```python
from build123d import *

# Parameters (mm, degrees)
ESQUISSE1_W                                  = 250
ESQUISSE1_H                                  = 400
BOSS_EXTRU_1_DEPTH                           = 10
ESQUISSE2_R                                  = 13.5
ENL_V_MAT_EXTRU_1_DEPTH                      = 237.061432682
CHANFREIN1_SIZE                              = 3
TROU_TARAUD_M51_D                            = 4.2
TROUS_DE_CENTRAGE_4_0MM2_D                   = 4
TROUS_DE_CENTRAGE_6_0MM2_D                   = 6
D_GAGEMENT_M41_D                             = 4.5
R_P_TITION_LIN_AIRE1_COUNT                   = 2
R_P_TITION_LIN_AIRE1_PITCH                   = 120
R_P_TITION_LIN_AIRE1_COUNT_DIR2              = 2
R_P_TITION_LIN_AIRE1_PITCH_DIR2              = 340
R_P_TITION_LIN_AIRE2_COUNT                   = 2
R_P_TITION_LIN_AIRE2_PITCH                   = 30
R_P_TITION_LIN_AIRE2_COUNT_DIR2              = 2
R_P_TITION_LIN_AIRE2_PITCH_DIR2              = 25
R_P_TITION_LIN_AIRE3_COUNT                   = 2
R_P_TITION_LIN_AIRE3_PITCH                   = 120
R_P_TITION_LIN_AIRE3_COUNT_DIR2              = 2
R_P_TITION_LIN_AIRE3_PITCH_DIR2              = 340
D_GAGEMENT_M42_D                             = 4.5
CHAMBRAGE_POUR_VIS_T_TE_RONDE_BOMB_2_A_COUNT = 2
CHAMBRAGE_POUR_VIS_T_TE_RONDE_BOMB_2_A_PITCH = 180
CHAMBRAGE_POUR_VIS_T_TE_RONDE_BOMB_3_COUNT   = 2
CHAMBRAGE_POUR_VIS_T_TE_RONDE_BOMB_3_PITCH   = 180
CHAMBRAGE_POUR_VIS_T_TE_RONDE_BOMB_4_COUNT   = 2
CHAMBRAGE_POUR_VIS_T_TE_RONDE_BOMB_4_PITCH   = 254.558441227
D_GAGEMENT_M43_D                             = 4.5
CHAMBRAGE_POUR_VIS_T_TE_RONDE_BOMB_5_A_COUNT = 2
CHAMBRAGE_POUR_VIS_T_TE_RONDE_BOMB_5_A_PITCH = 26.858717456
CUT_EXTRUDE1_DEPTH                           = 10


with BuildPart() as part:
    # Esquisse1 → Boss.-Extru.1 (new body)
    with BuildSketch(Plane.XY):
        Rectangle(ESQUISSE1_W, ESQUISSE1_H)
    extrude(amount=BOSS_EXTRU_1_DEPTH)

    # Esquisse2 → Enlèv. mat.-Extru.1 (cut, through all)
    with BuildSketch(Plane(origin=(0, 0, 0), x_dir=(-1, 0, 0), z_dir=(0, 0, -1))):
        Circle(ESQUISSE2_R)
    extrude(amount=-ENL_V_MAT_EXTRU_1_DEPTH, mode=Mode.SUBTRACT)

    # Chanfrein1
    chanfrein1_edges = [part.edges().sort_by_distance(p)[0] for p in [
        (125, -200, 5),
        (-125, -200, 5),
        (-125, 200, 5),
        (125, 200, 5),
    ]]
    chamfer(chanfrein1_edges, length=CHANFREIN1_SIZE)

    # Trou taraudé M51 (through all)
    with Locations(Plane.XY.offset(10)):
        with Locations((-72.698486264, -161.07971462), (-72.698486264, -181.838730229), (-111.937151978, -181.838730229), (-111.937151978, -161.07971462)):
            Hole(TROU_TARAUD_M51_D / 2)

    # Trous de centrage Ø4.0mm2 (through all)
    with Locations(Plane.XY.offset(10)):
        with Locations((-93.86308218, -161.07971462), (-93.86308218, -181.838730229)):
            Hole(TROUS_DE_CENTRAGE_4_0MM2_D / 2)

    # Trous de centrage Ø6.0mm2 (through all)
    with Locations(Plane.XY.offset(10)):
        with Locations((16.357059687, 37.86831259), (37.86831259, -16.357059687), (-16.357059687, -37.86831259), (-37.86831259, 16.357059687)):
            Hole(TROUS_DE_CENTRAGE_6_0MM2_D / 2)

    # Dégagement M41 (through all)
    with Locations(Plane(origin=(0, 0, 0), x_dir=(-1, 0, 0), z_dir=(0, 0, -1))):
        with Locations((28, -187), (28, -157), (53, -157), (53, -187)):
            d_gagement_m41 = Hole(D_GAGEMENT_M41_D / 2)

    # Répétition linéaire1: D_gagement M41 2 × 2
    with Locations(*[(i * R_P_TITION_LIN_AIRE1_PITCH, j * R_P_TITION_LIN_AIRE1_PITCH_DIR2, 0) for i in range(R_P_TITION_LIN_AIRE1_COUNT) for j in range(R_P_TITION_LIN_AIRE1_COUNT_DIR2) if (i, j) != (0, 0)]):
        add(d_gagement_m41, mode=Mode.SUBTRACT)

    # Esquisse29 → Chambrage pour vis _ t_te ronde bomb_e M (revolve, cut)
    with BuildSketch(Plane(origin=(92, -157, 10), x_dir=(0, -1, 0), z_dir=(1, 0, 0))):
        Polygon((0, 0), (0, 10), (2.25, 10), (2.25, 3.125), (2.275, 3.1), (4.5, 3.1), (4.5, 0), align=None)
    chambrage_pour_vis_t_te_ronde_bomb_e_m = revolve(axis=Axis((92, -157, 16.35), (0, 0, -1)), mode=Mode.SUBTRACT)

    # Répétition linéaire2: Chambrage pour vis _ t_te ronde bomb_e M 2 × 2
    with Locations(*[(-j * R_P_TITION_LIN_AIRE2_PITCH_DIR2, -i * R_P_TITION_LIN_AIRE2_PITCH, 0) for i in range(R_P_TITION_LIN_AIRE2_COUNT) for j in range(R_P_TITION_LIN_AIRE2_COUNT_DIR2) if (i, j) != (0, 0)]):
        add(chambrage_pour_vis_t_te_ronde_bomb_e_m, mode=Mode.SUBTRACT)

    # Répétition linéaire3: Chambrage pour vis _ t_te ronde bomb_e M 2 × 2
    with Locations(*[(-i * R_P_TITION_LIN_AIRE3_PITCH, j * R_P_TITION_LIN_AIRE3_PITCH_DIR2, 0) for i in range(R_P_TITION_LIN_AIRE3_COUNT) for j in range(R_P_TITION_LIN_AIRE3_COUNT_DIR2) if (i, j) != (0, 0)]):
        add(chambrage_pour_vis_t_te_ronde_bomb_e_m, mode=Mode.SUBTRACT)

    # Répétition linéaire3 copy 1 sketch → Répétition linéaire3 copy 1 (revolve, cut)
    with BuildSketch(Plane(origin=(67, 183, 10), x_dir=(0, -1, 0), z_dir=(1, 0, 0))):
        Polygon((0, 0), (0, 10), (2.25, 10), (2.25, 3.125), (2.275, 3.1), (4.5, 3.1), (4.5, 0), align=None)
    revolve(axis=Axis((67, 183, 16.35), (0, 0, -1)), mode=Mode.SUBTRACT)

    # Répétition linéaire3 copy 2 sketch → Répétition linéaire3 copy 2 (revolve, cut)
    with BuildSketch(Plane(origin=(-53, -157, 10), x_dir=(0, -1, 0), z_dir=(1, 0, 0))):
        Polygon((0, 0), (0, 10), (2.25, 10), (2.25, 3.125), (2.275, 3.1), (4.5, 3.1), (4.5, 0), align=None)
    revolve(axis=Axis((-53, -157, 16.35), (0, 0, -1)), mode=Mode.SUBTRACT)

    # Répétition linéaire3 copy 3 sketch → Répétition linéaire3 copy 3 (revolve, cut)
    with BuildSketch(Plane(origin=(-53, 183, 10), x_dir=(0, -1, 0), z_dir=(1, 0, 0))):
        Polygon((0, 0), (0, 10), (2.25, 10), (2.25, 3.125), (2.275, 3.1), (4.5, 3.1), (4.5, 0), align=None)
    revolve(axis=Axis((-53, 183, 16.35), (0, 0, -1)), mode=Mode.SUBTRACT)

    # Répétition linéaire3 copy 4 sketch → Répétition linéaire3 copy 4 (revolve, cut)
    with BuildSketch(Plane(origin=(92, 153, 10), x_dir=(0, -1, 0), z_dir=(1, 0, 0))):
        Polygon((0, 0), (0, 10), (2.25, 10), (2.25, 3.125), (2.275, 3.1), (4.5, 3.1), (4.5, 0), align=None)
    revolve(axis=Axis((92, 153, 16.35), (0, 0, -1)), mode=Mode.SUBTRACT)

    # Répétition linéaire3 copy 5 sketch → Répétition linéaire3 copy 5 (revolve, cut)
    with BuildSketch(Plane(origin=(-28, -187, 10), x_dir=(0, -1, 0), z_dir=(1, 0, 0))):
        Polygon((0, 0), (0, 10), (2.25, 10), (2.25, 3.125), (2.275, 3.1), (4.5, 3.1), (4.5, 0), align=None)
    revolve(axis=Axis((-28, -187, 16.35), (0, 0, -1)), mode=Mode.SUBTRACT)

    # Répétition linéaire3 copy 6 sketch → Répétition linéaire3 copy 6 (revolve, cut)
    with BuildSketch(Plane(origin=(-28, 153, 10), x_dir=(0, -1, 0), z_dir=(1, 0, 0))):
        Polygon((0, 0), (0, 10), (2.25, 10), (2.25, 3.125), (2.275, 3.1), (4.5, 3.1), (4.5, 0), align=None)
    revolve(axis=Axis((-28, 153, 16.35), (0, 0, -1)), mode=Mode.SUBTRACT)

    # Répétition linéaire3 copy 7 sketch → Répétition linéaire3 copy 7 (revolve, cut)
    with BuildSketch(Plane(origin=(67, 153, 10), x_dir=(0, -1, 0), z_dir=(1, 0, 0))):
        Polygon((0, 0), (0, 10), (2.25, 10), (2.25, 3.125), (2.275, 3.1), (4.5, 3.1), (4.5, 0), align=None)
    revolve(axis=Axis((67, 153, 16.35), (0, 0, -1)), mode=Mode.SUBTRACT)

    # Répétition linéaire3 copy 8 sketch → Répétition linéaire3 copy 8 (revolve, cut)
    with BuildSketch(Plane(origin=(-53, -187, 10), x_dir=(0, -1, 0), z_dir=(1, 0, 0))):
        Polygon((0, 0), (0, 10), (2.25, 10), (2.25, 3.125), (2.275, 3.1), (4.5, 3.1), (4.5, 0), align=None)
    revolve(axis=Axis((-53, -187, 16.35), (0, 0, -1)), mode=Mode.SUBTRACT)

    # Répétition linéaire3 copy 9 sketch → Répétition linéaire3 copy 9 (revolve, cut)
    with BuildSketch(Plane(origin=(-53, 153, 10), x_dir=(0, -1, 0), z_dir=(1, 0, 0))):
        Polygon((0, 0), (0, 10), (2.25, 10), (2.25, 3.125), (2.275, 3.1), (4.5, 3.1), (4.5, 0), align=None)
    revolve(axis=Axis((-53, 153, 16.35), (0, 0, -1)), mode=Mode.SUBTRACT)

    # Dégagement M42 (through all)
    with Locations(Plane(origin=(0, 0, 0), x_dir=(-1, 0, 0), z_dir=(0, 0, -1))):
        with Locations((90, -90), (90, 90), (-90, 90), (-90, -90)):
            Hole(D_GAGEMENT_M42_D / 2)

    # Esquisse33 → Chambrage pour vis _ t_te ronde bomb 2 (revolve, cut)
    with BuildSketch(Plane(origin=(-90, -90, 10), x_dir=(0, -1, 0), z_dir=(1, 0, 0))):
        Polygon((0, 0), (0, 10), (2.25, 10), (2.25, 3.125), (2.275, 3.1), (4.5, 3.1), (4.5, 0), align=None)
    chambrage_pour_vis_t_te_ronde_bomb_2 = revolve(axis=Axis((-90, -90, 16.35), (0, 0, -1)), mode=Mode.SUBTRACT)

    # Chambrage pour vis _ t_te ronde bomb 2 a: Chambrage pour vis _ t_te ronde bomb 2 ×2
    with Locations(*[(0, i * CHAMBRAGE_POUR_VIS_T_TE_RONDE_BOMB_2_A_PITCH, 0) for i in range(1, CHAMBRAGE_POUR_VIS_T_TE_RONDE_BOMB_2_A_COUNT)]):
        add(chambrage_pour_vis_t_te_ronde_bomb_2, mode=Mode.SUBTRACT)

    # Chambrage pour vis _ t_te ronde bomb 3: Chambrage pour vis _ t_te ronde bomb 2 ×2
    with Locations(*[(i * CHAMBRAGE_POUR_VIS_T_TE_RONDE_BOMB_3_PITCH, 0, 0) for i in range(1, CHAMBRAGE_POUR_VIS_T_TE_RONDE_BOMB_3_COUNT)]):
        add(chambrage_pour_vis_t_te_ronde_bomb_2, mode=Mode.SUBTRACT)

    # Chambrage pour vis _ t_te ronde bomb 4: Chambrage pour vis _ t_te ronde bomb 2 ×2
    with Locations(*[Vector(0.7071067811864814, 0.7071067811866137, 0) * (i * CHAMBRAGE_POUR_VIS_T_TE_RONDE_BOMB_4_PITCH) for i in range(1, CHAMBRAGE_POUR_VIS_T_TE_RONDE_BOMB_4_COUNT)]):
        add(chambrage_pour_vis_t_te_ronde_bomb_2, mode=Mode.SUBTRACT)

    # Dégagement M43 (through all)
    with Locations(Plane(origin=(0, 0, 0), x_dir=(-1, 0, 0), z_dir=(0, 0, -1))):
        with Locations((55.199022773, 135.70653433), (28.341819814, 135.991758108)):
            Hole(D_GAGEMENT_M43_D / 2)

    # Esquisse37 → Chambrage pour vis _ t_te ronde bomb 5 (revolve, cut)
    with BuildSketch(Plane(origin=(-55.199022773, 135.70653433, 10), x_dir=(0, -1, 0), z_dir=(1, 0, 0))):
        Polygon((0, 0), (0, 10), (2.25, 10), (2.25, 3.125), (2.275, 3.1), (4.5, 3.1), (4.5, 0), align=None)
    chambrage_pour_vis_t_te_ronde_bomb_5 = revolve(axis=Axis((-55.199022773, 135.70653433, 16.35), (0, 0, -1)), mode=Mode.SUBTRACT)

    # Chambrage pour vis _ t_te ronde bomb 5 a: Chambrage pour vis _ t_te ronde bomb 5 ×2
    with Locations(*[Vector(0.9999436124580966, 0.010619411671655749, 0) * (i * CHAMBRAGE_POUR_VIS_T_TE_RONDE_BOMB_5_A_PITCH) for i in range(1, CHAMBRAGE_POUR_VIS_T_TE_RONDE_BOMB_5_A_COUNT)]):
        add(chambrage_pour_vis_t_te_ronde_bomb_5, mode=Mode.SUBTRACT)

    # Sketch2 → Cut-Extrude1 (cut)
    with BuildSketch(Plane.XY.offset(10)):
        with BuildLine():
            Line((-104, 36), (-62, 36))
            ThreePointArc((-62, 36), (-59.171572875, 34.828427125), (-58, 32))
            Line((-58, 32), (-58, -30))
            ThreePointArc((-58, -30), (-59.171572875, -32.828427125), (-62, -34))
            Line((-62, -34), (-104, -34))
            ThreePointArc((-104, -34), (-106.828427125, -32.828427125), (-108, -30))
            Line((-108, -30), (-108, 32))
            ThreePointArc((-108, 32), (-106.828427125, 34.828427125), (-104, 36))
        make_face()
    extrude(amount=-CUT_EXTRUDE1_DEPTH, mode=Mode.SUBTRACT)


solid = part.part
```
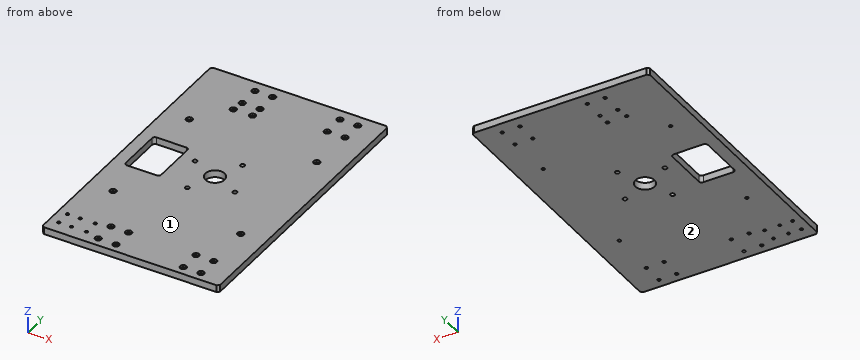
Read the model definition and answer for the solid it produces. Units are mm, in the model's axes. Face numbers are marked on the shaded views. Give positions to 0.01 mm unless a question says otherwise; leave off trailing zeros. Write each loop counter-clockwise with the first axis right and the second up, starting at its lowest first coordinate (ties: lowest second). Pieces come first, ordered by that corner, then holes. Notation, with made-up numbers: M -19.75,31 L 11.25,31 A28 cw 11.25,67 Z; hole C 24.5,84 d4. An arc over 180 degrees is marked long. Put each result on its own line as item: value. Start each with the question number.
1. Each of these flat-tipped pins is pushed along its axis until it touches: pin 1 Ø5.5 at (x, y) = (37.87, -16.36) entering from +Z; pin 2 Ø7 at (x, y) = (90, -90) entering from +Z. Where does it stop, or does it pass through?
2. The part is cut by section A-A, the plane y = 0. Give the vertices of the cut face in (x, z).
3. For a pull along Z with two mould halves and no side action, classify the marked faces 1 and 2 as released by +Z, released by -Z, zero draft, split by the parting line, or undercut.
4. Consider line 1 along X through (y, z) = (-157, 4); line 2 along X through (y, z) = (153, 8.7); line 3 along Y through (x, z) = (67, 7.75). Determine where each line is inside the solid, lowest interval first.
Final values:
1. pin 1: passes through
1. pin 2: stops at z = 6.9
2. outline: M -125,0 L -108,0 L -108,10 L -125,10 Z; M -58,0 L -13.5,0 L -13.5,10 L -58,10 Z; M 13.5,0 L 125,0 L 125,10 L 13.5,10 Z
3. face 1: released by +Z
3. face 2: released by -Z
4. line 1: x = -125 to -55.25, -50.75 to -30.25, -25.75 to 64.75, 69.25 to 89.75, 94.25 to 125
4. line 2: x = -125 to -57.5, -48.5 to -32.5, -23.5 to 62.5, 71.5 to 87.5, 96.5 to 125
4. line 3: y = -200 to -191.5, -182.5 to -161.5, -152.5 to 148.5, 157.5 to 178.5, 187.5 to 200
